Work out the finished part from the listing and answer in its coordinate system (mm). Face numbers are marked on the shaded views. A direction names the side the tool comes from. Round coordinates to 2 decimals unless told otherwise and drop trailing zeros. Loops run counter-clockwise (first coordinate to the right, second up) from the corner with the lowest first, then second, coordinate; pieces in that order, holes last. Notation, with made-up numbers: (-16.75, -5) - (42.25, -5) arc R31 cw to (42.25, 31) - close; hole circle Ø10 at (81.5, 24). An arc over 180 degrees is marked (long way). Return JSON: item names as keys, results as strings.
from build123d import *

# Parameters (mm, degrees)
F1_DEPTH  = 25.4
F3_DEPTH  = 127
F4_W      = 4.7752
F4_H      = 26.924
F5_DEPTH  = 50.8
F6_R      = 3.9751
F7_DEPTH  = 25.4
F8_W      = 26.924
F8_H      = 57.4802
F9_DEPTH  = 25.4
F10_W     = 21.8948
F10_H     = 26.924
F11_DEPTH = 3.9878


with BuildPart() as f1:
    # F0 (on Top) → F1 (new body)
    with BuildSketch(Plane.XY):
        Polygon((-74.295, 0), (0, 0), (0, 26.924), (-26.67, 26.924), (-26.67, 7.874), (-59.69, 7.874), (-59.69, 26.924), (-102.87, 26.924), (-102.87, 21.844), (-74.295, 21.844), align=None)
    extrude(amount=F1_DEPTH)

    # F2 (on face) → F3 (cut)
    with BuildSketch(Plane(origin=(0, 26.924, 0), x_dir=(-1, 0, 0), z_dir=(0, 1, 0))):
        with BuildLine():
            Line((90.17, 19.177), (90.17, 6.223))
            ThreePointArc((90.17, 6.223), (96.647, 12.7), (90.17, 19.177))
        make_face()
        with BuildLine():
            Line((83.82, 6.223), (90.17, 6.223))
            Line((90.17, 6.223), (90.17, 19.177))
            Line((90.17, 19.177), (83.82, 19.177))
            ThreePointArc((83.82, 19.177), (77.343, 12.7), (83.82, 6.223))
        make_face()
    extrude(amount=-F3_DEPTH, mode=Mode.SUBTRACT)

    # F4 (on face) → F5 (join)
    with BuildSketch(Plane.XY.offset(25.4)):
        with Locations((-24.2824, 13.462)):
            Rectangle(F4_W, F4_H)
    extrude(amount=F5_DEPTH)

    # F6 (on face) → F7 (cut)
    with BuildSketch(Plane(origin=(-26.67, 0, 0), x_dir=(0, -1, 0), z_dir=(-1, 0, 0))):
        with Locations((-12.7, 62.738)):
            Circle(F6_R)
    extrude(amount=-F7_DEPTH, mode=Mode.SUBTRACT)

    # F8 (on face) → F9 (cut)
    with BuildSketch(Plane.YZ.offset(-21.8948)):
        with Locations((13.462, 47.4599)):
            Rectangle(F8_W, F8_H)
    extrude(amount=F9_DEPTH, mode=Mode.SUBTRACT)

    # F10 (on face) → F11 (cut)
    with BuildSketch(Plane.XY.offset(18.7198)):
        with Locations((-10.9474, 13.462)):
            Rectangle(F10_W, F10_H)
    extrude(amount=-F11_DEPTH, mode=Mode.SUBTRACT)


solid = f1.part
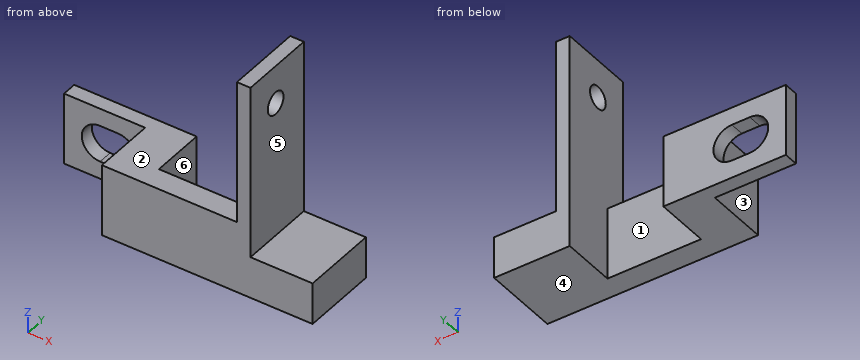
1) A tool of negligible diameter and unlimited length cuts with its end or side. For the marked faces 1, 2 and 3, from which of +Z, -Z, +X, -X, +Y, -Y can it reach the whole face along a straight path? Write none if from no direction.
Verdict:
{"face 1": "+Z, -Z, +Y", "face 2": "+Z, -X, +Y, -Y", "face 3": "+Z, -Z, -X, -Y"}
2) Section B-B (z = 12.7) is taken. Give the vertices of the cut face in (x, y) (3 decimals).
Verdict:
{"outline": "(-102.87, 21.844) - (-96.647, 21.844) - (-96.647, 26.924) - (-102.87, 26.924) - close; (-77.343, 21.844) - (-74.295, 21.844) - (-74.295, 0) - (0, 0) - (0, 26.924) - (-26.67, 26.924) - (-26.67, 7.874) - (-59.69, 7.874) - (-59.69, 26.924) - (-77.343, 26.924) - close"}
3) Flat-ended cylindrical pins translate along their axes: pin 1 (6.5 mm diameter, centred on x = -13, y = 15.5, fed in from +Z); pin 2 (3 mm diameter, centred on y = 17.5, z = 41, fed in from -X); pin 3 (2.5 mm diameter, centred on x = -86.5, y = 24, fed in from +Z). Find the tip coordinate at first contact, or state that the pin passes through.
Verdict:
{"pin 1": "stops at z = 14.73", "pin 2": "stops at x = -26.67", "pin 3": "stops at z = 25.4"}
4) Determine the mould class of the marked faces 4, 5 and 6 for opening direction X: pulls with the +X half, pulls with the -X half, needs draft (parallel to the pull), parting line crosses it, or undercut.
Verdict:
{"face 4": "needs draft", "face 5": "pulls with the +X half", "face 6": "undercut"}
5) Section D-D (z = 31) is taken. Give the vertices of the cut face in (x, y).
Verdict:
{"outline": "(-26.67, 0) - (-21.89, 0) - (-21.89, 26.92) - (-26.67, 26.92) - close"}
6) Section A-A (y = 12.7) is taken. Give the vertices of the cut face in (x, z) (3 decimals).
Verdict:
{"outline": "(-74.295, 0) - (-59.69, 0) - (-59.69, 25.4) - (-74.295, 25.4) - close; (-26.67, 0) - (0, 0) - (0, 14.732) - (-21.895, 14.732) - (-21.895, 58.763) - (-26.67, 58.763) - close; (-26.67, 66.713) - (-21.895, 66.713) - (-21.895, 76.2) - (-26.67, 76.2) - close"}
7) Find the intervals of material crossed by L1, parallel to X at y = 17, z = 4 (3 decimals); L2, parallel to Z at x = -25.3, y = 12.7; L3, parallel to X at y = 24.75, z = 24, in increasing order.
Verdict:
{"L1": "x = -74.295 to -59.69, -26.67 to 0", "L2": "z = 0 to 58.76, 66.71 to 76.2", "L3": "x = -102.87 to -59.69, -26.67 to -21.89"}
8) Section C-C (x = -82.5) is taken. Give the vertices of the cut face in (y, z), and give its area (3 significant figures).
Verdict:
{"outline": "(21.84, 0) - (26.92, 0) - (26.92, 6.36) - (21.84, 6.36) - close; (21.84, 19.04) - (26.92, 19.04) - (26.92, 25.4) - (21.84, 25.4) - close", "area": "64.6 mm2"}
